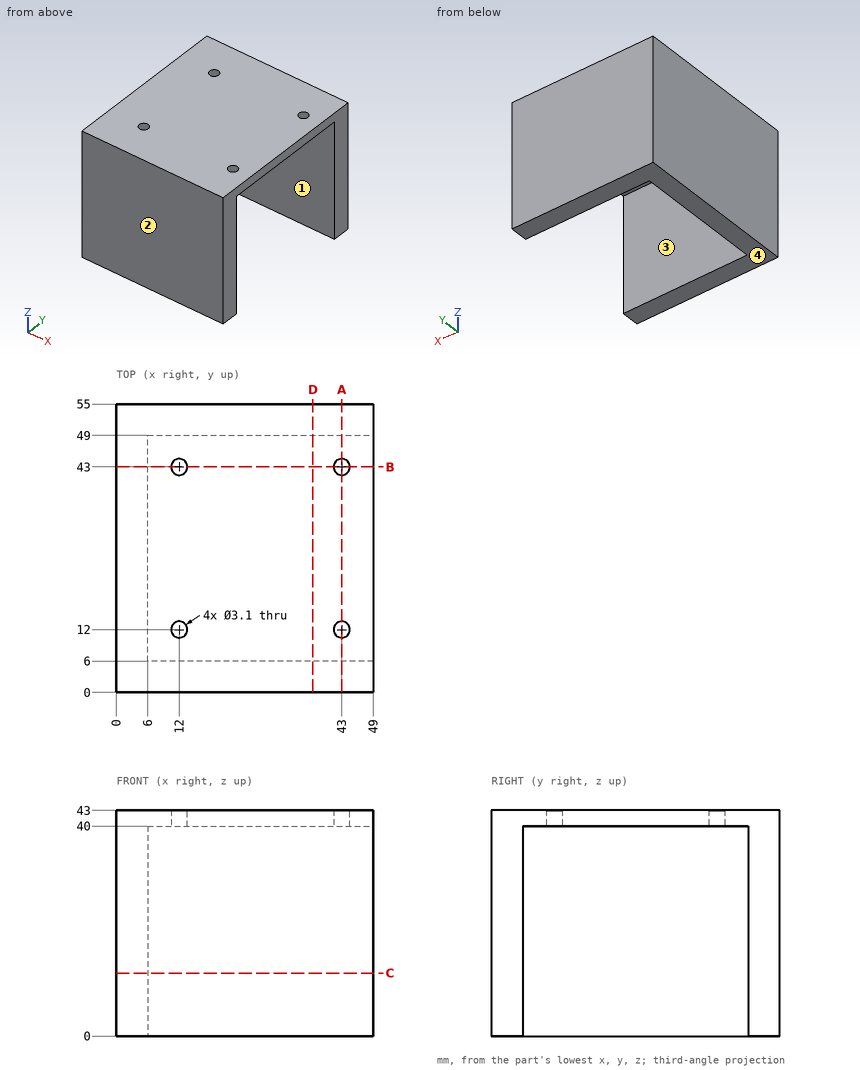
Geometry check sheet. Reference: drawing and pictorial views, mm from the part's lowest x, y, z. Round coordinates to 2 decimals unless told otherwise and drop trailing zeros. Order: outer loops, then holes, each group sorted by start corner. A loop starts at its lowest first (then second) coordinate and runs counter-clockwise, first axis right, second up. Notation, with made-up numbers: (-13, 35) - (22, 35) arc R14 ccw to (22, 55) - close; hole circle Ø4 at (47.5, -3). An arc over 180 degrees is marked (long way). Use a Markdown table: item, result. Add a question column.
1) Gauge pin test, flat ends, axial feed: P1, Ø1, axis at x = 19, y = 8, coming from the -Z side; P2, Ø12, axis at y = 34, z = 27.5, coming from the +X side. Record the tip position at first contact, or that the pin passes through.
2) Section check A-A (x = 43). Record the cut outline in (y, z).
3) Thickness scan on line 1 along Y through (x, z) = (12, 42); line 2 along Y through (x, z) = (43, 24.5); line 3 along Z through (x, y) = (22.5, 35.5). Record the ranges inside material, lowest first.
4) Mould release check, pull along Y, two halves, no side actions. Record for the marked faces 1, 2, 3 and 4: released by +Y, released by -Y, zero draft, split by the parting line, or undercut.
5) Section check B-B (y = 43). Record the cut outline in (x, z).
6) Section check D-D (x = 37.5). Record the cut outline in (y, z), then the cut area to 3 significant figures.
7) Section check C-C (z = 12). Record the cut outline in (x, y).
Established:
| question | item | result |
|---|---|---|
| 1 | P1 | z = 40 |
| 1 | P2 | x = 6 |
| 2 | outline | (0, 0) - (6, 0) - (6, 40) - (10.45, 40) - (10.45, 43) - (0, 43) - close; (13.55, 40) - (41.45, 40) - (41.45, 43) - (13.55, 43) - close; (44.55, 40) - (49, 40) - (49, 0) - (55, 0) - (55, 43) - (44.55, 43) - close |
| 3 | line 1 | 0 to 10.45, 13.55 to 41.45, 44.55 to 55 |
| 3 | line 2 | 0 to 6, 49 to 55 |
| 3 | line 3 | 40 to 43 |
| 4 | face 1 | undercut |
| 4 | face 2 | released by -Y |
| 4 | face 3 | undercut |
| 4 | face 4 | zero draft |
| 5 | outline | (0, 0) - (6, 0) - (6, 40) - (10.45, 40) - (10.45, 43) - (0, 43) - close; (13.55, 40) - (41.45, 40) - (41.45, 43) - (13.55, 43) - close; (44.55, 40) - (49, 40) - (49, 43) - (44.55, 43) - close |
| 6 | outline | (0, 0) - (6, 0) - (6, 40) - (49, 40) - (49, 0) - (55, 0) - (55, 43) - (0, 43) - close |
| 6 | area | 645 mm2 |
| 7 | outline | (0, 0) - (49, 0) - (49, 6) - (6, 6) - (6, 49) - (49, 49) - (49, 55) - (0, 55) - close |
